Build history of the part. All positions in model axes, mm. A direction names the side the tool comes from. Round coordinates to 2 decimals unless told otherwise and drop trailing zeros. Write each loop counter-clockwise with the first axis right and the second up, starting at its lowest first coordinate (ties: lowest second). Pieces come first, ordered by that corner, then holes.
1) Pull direction X, two halves, no side cores. Call faces 1 (the flat face through (0, 9, 2)), 2 (the flat face through (25, 0, 2)), 3 (the cylindrical face through (37.547, 10.208, 1.565)): +X half, -X half, draft (parallel to the pull), parting line (faces both ways), or undercut.
2) Saw through at D-D (x = 1). Write the cut outline in (y, z) (3 decimals).
3) Saw through at A-A (x = 12.7). Write the cut outline in (y, z) (3 decimals).
4) Which spindle directions (+Z, -Z, +X, -X, +Y, -Y) get a long thin tool onto all of the face, cutting with end or side? Do faces 4 (the cylindrical face through (-8.88, 44.51, 1.57)), 5 (the cylindrical face through (-34.7, 49.8, 1.6)), 6 (the flat face through (-18, 19.05, 2)). Say none if no direction does.
5) Saw through at B-B (z = 1.7). Write the cut outline in (x, y) (3 decimals), plus the area to 3 significant figures.
6) Saw through at C-C (y = 27). Write the cut outline in (x, z) (3 decimals), plus the area to 3 significant figures.
7) Flat gauge pin, fed straight in: pin 1 (3 mm diameter, centred on x = -11.43, y = 25.4, fed in from +Z). Where does the tip first touch, or does it go through?
8) Wall check: probe 1 along Y at (x, z) = (12.7, 1.9); probe 2 along X at (y, z) = (3, 1.8); probe 3 along Y at (x, z) = (-27, 1.65). Give the ranges that are in metal, low to high.
from build123d import *

# Parameters (mm, degrees)
SKETCH1_W           = 50.8
SKETCH1_H           = 50.8
SKETCH1_R           = 2.5527
SKETCH1_W_2         = 35.56
SKETCH1_H_2         = 31.75
BOSS_EXTRUDE1_DEPTH = 3.175
FILLET1_R           = 3.175


with BuildPart() as part:
    # Sketch1 → Boss-Extrude1 (new body)
    # profile 1 of 2: a face of its own
    with BuildSketch(Plane.XY):
        with Locations((25.4, 25.4)):
            Rectangle(SKETCH1_W, SKETCH1_H)
        with Locations((38.1, 12.7)):
            Circle(SKETCH1_R, mode=Mode.SUBTRACT)
        with Locations((12.7, 12.7)):
            Circle(SKETCH1_R, mode=Mode.SUBTRACT)
    # profile 2 of 2: a face of its own
    with BuildSketch(Plane.XY):
        with Locations((-17.78, 34.925)):
            Rectangle(SKETCH1_W_2, SKETCH1_H_2)
        with Locations((-11.43, 25.4)):
            Circle(SKETCH1_R, mode=Mode.SUBTRACT)
        with BuildLine():
            ThreePointArc((-25.717080894, 33.64865), (-29.204133942, 32.714296952), (-30.13848699, 36.20135))
            ThreePointArc((-30.13848699, 36.20135), (-22.23135, 44.10848699), (-11.43, 47.0027))
            ThreePointArc((-11.43, 47.0027), (-8.8773, 44.45), (-11.43, 41.8973))
            ThreePointArc((-11.43, 41.8973), (-19.67865, 39.687080894), (-25.717080894, 33.64865))
        make_face(mode=Mode.SUBTRACT)
    extrude(amount=BOSS_EXTRUDE1_DEPTH)

    # Fillet1
    fillet1_edges = [part.edges().sort_by_distance(p)[0] for p in [
        (0, 0, 1.5875),
        (0, 19.05, 1.5875),
        (-35.56, 19.05, 1.5875),
        (-35.56, 50.8, 1.5875),
        (50.8, 50.8, 1.5875),
        (50.8, 0, 1.5875),
    ]]
    fillet(fillet1_edges, radius=FILLET1_R)


solid = part.part
Evaluation:
1. face 1: -X half
1. face 2: draft
1. face 3: undercut
2. outline: (0.862, 0) - (50.8, 0) - (50.8, 3.175) - (0.862, 3.175) - close
3. outline: (0, 0) - (10.147, 0) - (10.147, 3.175) - (0, 3.175) - close; (15.253, 0) - (50.8, 0) - (50.8, 3.175) - (15.253, 3.175) - close
4. face 4: +Z, -Z
4. face 5: +Z, -Z, -X, +Y
4. face 6: +Z, -Z, -X, -Y
5. outline: (-35.56, 22.225) arc R3.175 ccw to (-32.385, 19.05) - (-3.175, 19.05) arc R3.175 cw to (0, 15.875) - (0, 3.175) arc R3.175 ccw to (3.175, 0) - (47.625, 0) arc R3.175 ccw to (50.8, 3.175) - (50.8, 47.625) arc R3.175 ccw to (47.625, 50.8) - (-32.385, 50.8) arc R3.175 ccw to (-35.56, 47.625) - close; hole (-30.138, 36.201) arc R2.553 ccw to (-25.717, 33.649) arc R16.497 cw to (-11.43, 41.897) arc R2.553 ccw to (-11.43, 47.003) arc R21.603 ccw to start; hole circle Ø5.105 at (-11.43, 25.4); hole circle Ø5.105 at (12.7, 12.7); hole circle Ø5.105 at (38.1, 12.7)
5. area: 3,520 mm2
6. outline: (-35.56, 0) - (-13.419, 0) - (-13.419, 3.175) - (-35.56, 3.175) - close; (-9.441, 0) - (50.8, 0) - (50.8, 3.175) - (-9.441, 3.175) - close
6. area: 262 mm2
7. pin 1: passes through
8. probe 1: y = 0 to 10.15, 15.25 to 50.8
8. probe 2: x = 0 to 50.8
8. probe 3: y = 19.05 to 32.55, 40.38 to 50.8
